```python
from build123d import *

# Parameters (mm, degrees)
F1_DEPTH = 5


with BuildPart() as f1:
    # F0 (on Top) → F1 (new body)
    with BuildSketch(Plane.XY):
        with BuildLine():
            Line((-10, -3), (10, -3))
            Line((10, -3), (10, -0.25))
            Line((10, -0.25), (8.433013, -0.25))
            ThreePointArc((8.433013, -0.25), (7.5, 0), (8.433013, 0.25))
            Line((8.433013, 0.25), (10, 0.25))
            Line((10, 0.25), (10, 3))
            Line((10, 3), (-10, 3))
            Line((-10, 3), (-10, -3))
        make_face()
    extrude(amount=F1_DEPTH)


solid = f1.part
```
Geometry: final body of the model. Coordinates: model frame, mm. A direction names the side the tool comes from. Coordinates: 2 decimals unless noted, no trailing zeros. Order: outer loops, then holes, each group sorted by start corner. A loop starts at its lowest first (then second) coordinate and runs counter-clockwise, first axis right, second up. Notation, with made-up numbers: (4, -5.5) - (17, -5.5) arc R15 ccw to (17, 20.5) - close; hole circle Ø8 at (-26.75, 26). An arc over 180 degrees is marked (long way). Return JSON: item names as keys, results as strings. Group by question number.
1. Pull-direction query (X, two-part tool) for faces 3 (the face through (0, 0, 0)), 4 (the face through (-10, 0, 2)), 5 (the face through (10, 2, 2)), 6 (the face through (7.5, 0, 2.5)); classes: pulls with the +X half, pulls with the -X half, needs draft (parallel to the pull), parting line crosses it, or undercut.
2. Material intervals for line 1 along X through (y, z) = (0, 2.35); line 2 along X through (y, z) = (0.4, 2.5), sorted ascending. Write a range as [from, to].
3. Cut plane B-B (y = 0). Output: boundary loops of the cut face in (x, z).
4. Cut plane A-A (x = 8). Output: boundary loops of the cut face in (y, z), plus the area to 3 significant figures.
5. Set-up query: faces 1 (the face through (9, -0.25, 2)), 2 (the face through (0, 0, 5)). Return all of +Z, -Z, +X, -X, +Y, -Y with unobstructed straight access to the full face (end or side cutting, diameter ignored); none if empty.
6. Pin query (flat end, axial travel): pin 1 (0.6 mm diameter, centred on x = 8, y = 0, fed in from -Z). Return the tip coordinate at first contact, or that it passes through.
Resolved:
{
 "1": {"face 3": "needs draft", "face 4": "pulls with the -X half", "face 5": "pulls with the +X half", "face 6": "undercut"},
 "2": {"line 1": "x = [-10, 7.5]", "line 2": "x = [-10, 7.7], [8.3, 10]"},
 "3": {"outline": "(-10, 0) - (7.5, 0) - (7.5, 5) - (-10, 5) - close"},
 "4": {"outline": "(-3, 0) - (-0.5, 0) - (-0.5, 5) - (-3, 5) - close; (0.5, 0) - (3, 0) - (3, 5) - (0.5, 5) - close", "area": "25.0 mm²"},
 "5": {"face 1": "+Z, -Z, +X", "face 2": "+Z, +X, -X, +Y, -Y"},
 "6": {"pin 1": "passes through"}
}
